Autodesk Inventor part; units mm, degrees
ref_plane "YZ Plane" through (0, 0, 0) normal (1, 0, 0) x (0, 1, 0)
ref_plane "XZ Plane" through (0, 0, 0) normal (0, 1, 0) x (-1, 0, 0)
ref_plane "XY Plane" through (0, 0, 0) normal (0, 0, 1) x (1, 0, 0)
sketch "Sketch1" plane through (0, 0, 0) normal (0, 1, 0) x (-1, 0, 0)
  circle A0 centre (0, 0) radius 12.5
  arc A1 (25, 0) -> (-25, 0) centre (0, 0) ccw
  line L0 (-25, 0) -> (-25, -60)
  line L1 (-25, -60) -> (25, -60)
  line L2 (25, -60) -> (25, 0)
  dimension "d0" = 25
  dimension "d1" = 50
  dimension "d2" = 60
extrude "Extrusion1" add sketch "Sketch1" along normal blind 5
sketch "Sketch2" plane through (25, 0, -60) normal (0, 0, -1) x (-1, 0, 0)
  point P0 (25, 0)
sketch "Sketch3" plane through (25, 0, -60) normal (0, 0, -1) x (-1, 0, 0)
  line L0 (0, 0) -> (50, 0)
  line L1 (50, 0) -> (50, 30)
  line L2 (50, 30) -> (0, 30)
  line L3 (0, 30) -> (0, 0)
  point P0 (25, 0)
  dimension "d5" = 30
extrude "Extrusion2" add sketch "Sketch3" along normal blind 5
hole "Hole1" at (-10, 17.5, -60) direction (0, 0, -1) diameter 3 end through all
hole "Hole2" at (10, 17.5, -60) direction (0, 0, -1) diameter 3 end through all
fillet "Fillet1" radius 1 1 edges at (10, 19, -60)
fillet "Fillet2" radius 1 1 edges at (-10, 19, -60)
fillet "Fillet3" radius 1 2 edges at (12.5, 5, 0) (12.5, 0, 0)
fillet "Fillet4" radius 1 9 edges at (25, 5, -30) (-25, 5, -30) (0, 5, 25) (25, 17.5, -60) (-25, 17.5, -60) (0, 30, -60) (0, 0, 25) (-25, 0, -32.5) (25, 0, -32.5)
sketch "Sketch4" plane through (0, 0, 0) normal (0, -1, 0) x (1, 0, 0)
  circle A0 centre (0, 0) radius 17.7289
extrude "Extrusion3" add sketch "Sketch4" against normal blind 1.5
properties part number "Shop Towel Holder"
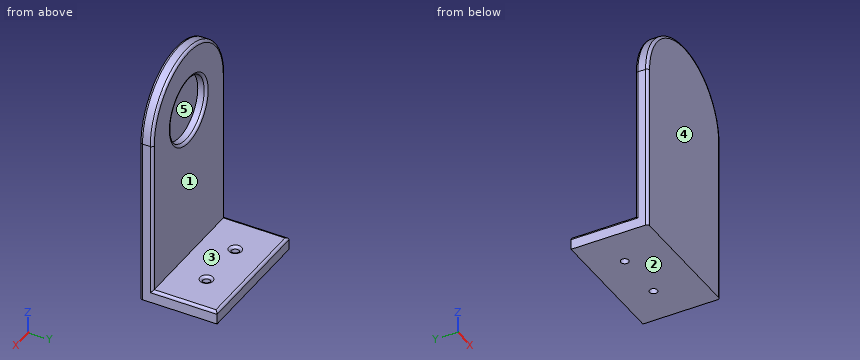
For this review, take the finished solid that the model builds, in its own axes (mm). Face numbers are marked on the shaded views. A direction names the side the tool comes from. Round coordinates to 2 decimals unless told otherwise and drop trailing zeros. Order: outer loops, then holes, each group sorted by start corner. A loop starts at its lowest first (then second) coordinate and runs counter-clockwise, first axis right, second up.
Q1. Machinability: for the marked faces 1 and 2, which of the approach directions +Z, -Z, +X, -X, +Y, -Y give a long, thin tool a straight path to every point of the face, cutting with its end or side? Answer none if there is none.
Findings below:
face 1: +Z, +X, -X, +Y
face 2: -Z, +X, -X, +Y, -Y
Q2. Insertion check: P1, Ø4, axis at x = 13.5, z = -35, coming from the -Y side; P2, Ø1, axis at x = -9.5, y = 22, coming from the +Z side; P3, Ø4, axis at x = -5, z = -23, coming from the +Y side; P4, Ø12.5, axis at x = 1.5, z = 2, coming from the +Y side. Each pin has a flat end and moves straight along its axis. Give the tip position at first contact, or say it passes through.
Findings below:
P1: stops at y = 0
P2: stops at z = -60
P3: stops at y = 5
P4: stops at y = 1.5
Q3. Mouldability with a two-part tool opening along Z and no side actions: class the marked faces 3, 4 and 5 as pulls with the +Z half, pulls with the -Z half, needs draft (parallel to the pull), parting line crosses it, or undercut.
Findings below:
face 3: pulls with the +Z half
face 4: needs draft
face 5: undercut
Q4. We need section B-B, the plane x = 0. Give the boundary of the cut face in (y, z).
Findings below:
outline: (0, -65) - (30, -65) - (30, -61) arc R1 ccw to (29, -60) - (5, -60) - (5, -13.5) arc R1 ccw to (4, -12.5) - (1.5, -12.5) - (1.5, 12.5) - (4, 12.5) arc R1 ccw to (5, 13.5) - (5, 24) arc R1 ccw to (4, 25) - (1, 25) arc R1 ccw to (0, 24) - close
Q5. We need section C-C, the plane y = 12. Give the boundary of the cut face in (x, z).
Findings below:
outline: (-25, -65) - (25, -65) - (25, -61) arc R1 ccw to (24, -60) - (-24, -60) arc R1 ccw to (-25, -61) - close
Q6. Wall thickness on line 1 (X direction, y = 17.5, z = -62.1); line 2 (Y direction, x = -10, z = -64.1); line 3 (Z direction, x = -9, y = 25): over which ranges is each line inside the solid? List them lowest first.
Findings below:
line 1: x = -25 to -11.5, -8.5 to 8.5, 11.5 to 25
line 2: y = 0 to 16, 19 to 30
line 3: z = -65 to -60
Q7. We need section A-A, the plane z = -56.5. Give the boundary of the cut face in (x, y), plus the area to 3 significant figures.
Findings below:
outline: (-25, 1) arc R1 ccw to (-24, 0) - (24, 0) arc R1 ccw to (25, 1) - (25, 4) arc R1 ccw to (24, 5) - (-24, 5) arc R1 ccw to (-25, 4) - close
area: 249 mm2
